Check sheet for the drawn part. Datum: minimum x, y, z corner. Units: mm. A direction names the side the tool comes from. Give positions to 0.01 mm unless a question says otherwise; leave off trailing zeros. Loops run counter-clockwise (first coordinate to the right, second up) from the corner with the lowest first, then second, coordinate; pieces in that order, holes last. Notation, with made-up numbers: (42.5, -29.75) - (66.5, -29.75) arc R9 cw to (66.5, -15.75) - close; hole circle Ø9 at (-37.75, 9.5). An arc over 180 degrees is marked (long way). Answer in a Markdown table with one row per item.
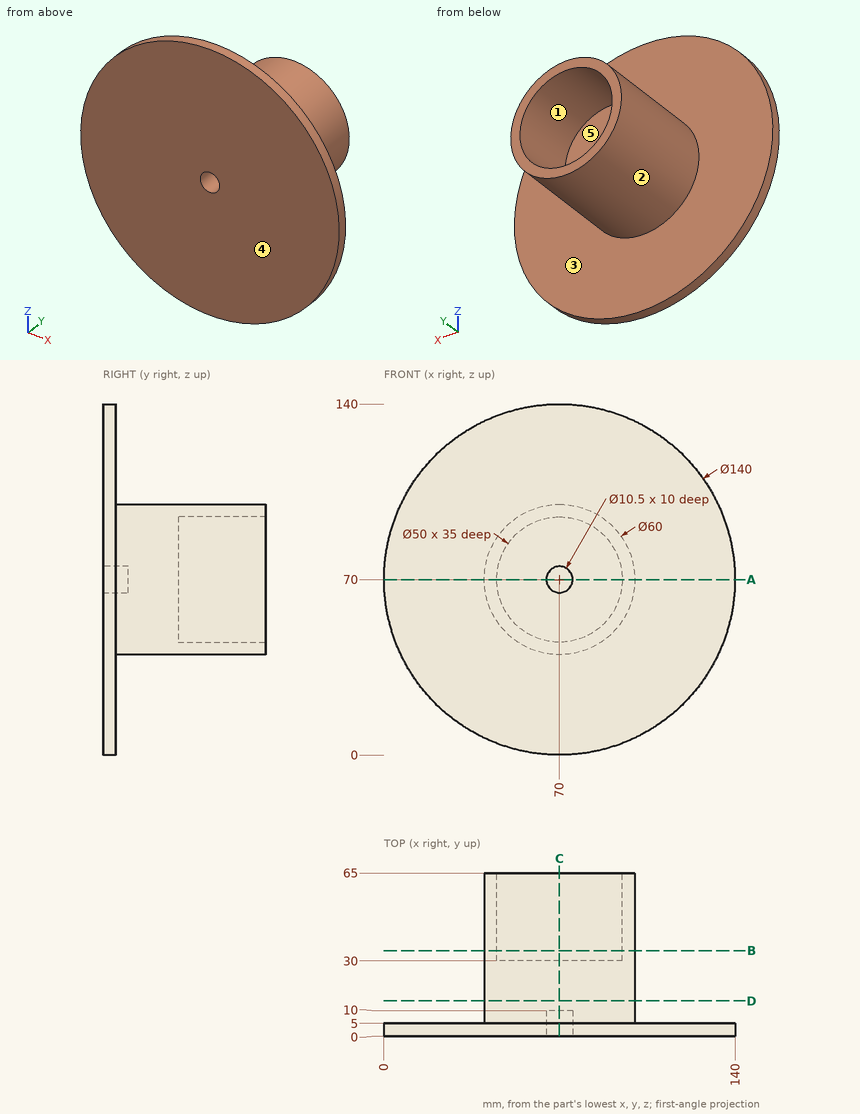
Q1. Thickness scan on line 1 (X direction, y = 56, z = 70); line 2 (Z direction, x = 70.5, y = 11); line 3 (Y direction, x = 84, z = 123). Record the ranges inside material, lowest first.
Completed:
| item | result |
|---|---|
| line 1 | 40 to 45, 95 to 100 |
| line 2 | 40 to 100 |
| line 3 | 0 to 5 |
Q2. Tool access check on the marked faces 4 and 5. Record the directions out of +Z, -Z, +X, -X, +Y, -Y that give a thin tool (end or side, any length) a straight path to the whole face; none if there is none.
Completed:
| item | result |
|---|---|
| face 4 | +Z, -Z, +X, -X, -Y |
| face 5 | +Y |
Q3. Sectioned sample at B-B (y = 34). Record the cut outline in (x, z), and give its area (3 significant figures).
Completed:
| item | result |
|---|---|
| outline | circle Ø60 at (70, 70); hole circle Ø50 at (70, 70) |
| area | 864 mm^2 |
Q4. Go/stop test with flat-tipped pins: P1, Ø25, axis at x = 76.5, z = 76.5, coming from the +Y side; P2, Ø1, axis at y = 49, z = 47.5, coming from the -X side; P3, Ø5, axis at x = 85.5, z = 35.5, coming from the +Y side. Record where each tip stops, or that it passes through.
Completed:
| item | result |
|---|---|
| P1 | y = 30 |
| P2 | x = 49.6 |
| P3 | y = 5 |
Q5. Sectioned sample at C-C (x = 70). Record the cut outline in (y, z).
Completed:
| item | result |
|---|---|
| outline | (0, 0) - (5, 0) - (5, 40) - (65, 40) - (65, 45) - (30, 45) - (30, 95) - (65, 95) - (65, 100) - (5, 100) - (5, 140) - (0, 140) - (0, 75.25) - (10, 75.25) - (10, 64.75) - (0, 64.75) - close |
Q6. Sectioned sample at A-A (z = 70). Record the cut outline in (x, y).
Completed:
| item | result |
|---|---|
| outline | (0, 0) - (64.75, 0) - (64.75, 10) - (75.25, 10) - (75.25, 0) - (140, 0) - (140, 5) - (100, 5) - (100, 65) - (95, 65) - (95, 30) - (45, 30) - (45, 65) - (40, 65) - (40, 5) - (0, 5) - close |
Q7. Draft check along Z on the marked faces 1, 2 and 3. Enter one of: +Z half, -Z half, draft (parallel to the pull), parting line (faces both ways), or undercut.
Completed:
| item | result |
|---|---|
| face 1 | undercut |
| face 2 | parting line |
| face 3 | draft |
Q8. Sectioned sample at D-D (y = 14). Record the cut outline in (x, z).
Completed:
| item | result |
|---|---|
| outline | circle Ø60 at (70, 70) |
